Autodesk Inventor part; units mm, degrees
ref_plane "YZ Plane" through (0, 0, 0) normal (1, 0, 0) x (0, 1, 0)
ref_plane "XZ Plane" through (0, 0, 0) normal (0, 1, 0) x (-1, 0, 0)
ref_plane "XY Plane" through (0, 0, 0) normal (0, 0, 1) x (1, 0, 0)
sketch "スケッチ1" plane through (0, 0, 0) normal (0, 0, 1) x (1, 0, 0)
  circle A0 centre (-490.19, 90.19) radius 2.1
  circle A1 centre (-490.19, 290.19) radius 2.1
  circle A2 centre (-190.19, 390.19) radius 2.1
  circle A3 centre (-390.19, 390.19) radius 2.1
  circle A4 centre (-290.19, -9.81) radius 2.1
  circle A5 centre (-90.19, -9.81) radius 2.1
  circle A6 centre (9.81, 190.19) radius 2.1
  circle A7 centre (9.81, 390.19) radius 2.1
  circle A8 centre (-490.19, -9.81) radius 2.1
  circle A9 centre (-233.68, 12.7) radius 1.6 construction
  circle A10 centre (-29.21, 294.64) radius 1.6 construction
  circle A11 centre (-161.29, 294.64) radius 1.6 construction
  circle A12 centre (-233.68, 294.64) radius 1.6 construction
  circle A13 centre (-233.68, 137.16) radius 1.6 construction
  circle A14 centre (-161.29, 137.16) radius 1.6 construction
  circle A15 centre (-6.35, 137.16) radius 1.6 construction
  circle A16 centre (-6.35, 12.7) radius 1.6 construction
  circle A17 centre (-161.29, 12.7) radius 1.6 construction
  circle A18 centre (9.81, -9.81) radius 2.1
  circle A19 centre (-490.19, 390.19) radius 2.1
  circle A20 centre (9.81, 290.19) radius 2.1
  circle A21 centre (9.81, 90.19) radius 2.1
  circle A22 centre (-190.19, -9.81) radius 2.1
  circle A23 centre (-390.19, -9.81) radius 2.1
  circle A24 centre (-290.19, 390.19) radius 2.1
  circle A25 centre (-90.19, 390.19) radius 2.1
  circle A26 centre (-490.19, 190.19) radius 2.1
  line L0 (-21.19, 1.19) -> (-459.19, 1.19)
  line L1 (-479.19, 21.19) -> (-479.19, 359.19)
  line L2 (-459.19, 379.19) -> (-21.19, 379.19)
  line L3 (-1.19, 359.19) -> (-1.19, 21.19)
  circle A27 centre (9.81, -9.81) radius 5
  circle A28 centre (9.81, -9.81) radius 15.5563 construction
  line L4 (9.81, -9.81) -> (-1.19, 1.19) construction
  line L5 (9.81, -9.81) -> (25.3663, -9.81) construction
  circle A29 centre (-1.19, 1.19) radius 5 construction
  circle A30 centre (-1.19, 1.19) radius 2.1
  line L6 (-240.19, 1.19) -> (-240.19, 379.19) construction
  line L7 (-1.19, 190.19) -> (-479.19, 190.19) construction
  circle A31 centre (-1.19, 379.19) radius 2.1
  circle A32 centre (-479.19, 1.19) radius 2.1
  circle A33 centre (-479.19, 379.19) radius 2.1
  arc A34 (-1.19, 359.19) -> (-21.19, 379.19) centre (-21.19, 359.19) ccw
  arc A35 (-459.19, 379.19) -> (-479.19, 359.19) centre (-459.19, 359.19) ccw
  arc A36 (-479.19, 21.19) -> (-459.19, 1.19) centre (-459.19, 21.19) ccw
  arc A37 (-21.19, 1.19) -> (-1.19, 21.19) centre (-21.19, 21.19) ccw
  line L8 (9.81, -4.81) -> (-11.2166, -4.81) construction
  arc A38 (-483.7257, 425.19) -> (-483.7257, -44.81) centre (161.4767, 190.19) ccw
  line L9 (-483.7257, 425.19) -> (-379.99, 425.19)
  arc A39 (-379.99, 425.19) -> (-100.39, 425.19) centre (-240.19, 735.924) ccw
  line L10 (-100.39, 425.19) -> (3.3457, 425.19)
  arc A40 (3.3457, -44.81) -> (3.3457, 425.19) centre (-641.8567, 190.19) ccw
  line L11 (3.3457, -44.81) -> (-79.99, -44.81)
  arc A41 (-79.99, -44.81) -> (-400.39, -44.81) centre (-240.19, -457.544) ccw
  line L12 (-400.39, -44.81) -> (-483.7257, -44.81)
  arc A42 (14.81, 390.19) -> (9.81, 395.19) centre (9.81, 390.19) ccw
  line L13 (9.81, 395.19) -> (-490.19, 395.19)
  line L14 (14.81, -9.81) -> (14.81, 390.19)
  arc A43 (9.81, -14.81) -> (14.81, -9.81) centre (9.81, -9.81) ccw construction
  line L15 (-490.19, -14.81) -> (9.81, -14.81)
  arc A44 (-495.19, -9.81) -> (-490.19, -14.81) centre (-490.19, -9.81) ccw
  line L16 (-495.19, 390.19) -> (-495.19, -9.81)
  arc A45 (-490.19, 395.19) -> (-495.19, 390.19) centre (-490.19, 390.19) ccw
  point P0 (0, 0)
  point P1 (-1.19, 1.19)
  point P2 (-479.19, 379.19)
  point P3 (-479.19, 1.19)
  point P4 (-1.19, 379.19)
  point P5 (14.59, -11.277)
  point P6 (-494.97, 391.657)
  point P7 (-494.97, -11.277)
  dimension "d4" = 31.1127
  dimension "d5" = 135
  dimension "d6" = 10
  dimension "d10" = 20
  dimension "d11" = 6
  dimension "d14" = 11
  dimension "d15" = 11
  dimension "d16" = 11
  dimension "d17" = 11
  dimension "d18" = 11
  dimension "d30" = 100
extrude "押し出し1" add sketch "スケッチ1" against normal blind 3 contours A27 | A27 L15 A44 L16 A45 L13 A42 L14 | A27 A40 L11 A41 L15 | A41 L12 A38 A44 L15 | A30 | A32
sketch "スケッチ3" plane through (0, 0, -3) normal (0, 0, -1) x (-1, 0, 0)
  arc A0 (-14.81, -9.81) -> (-14.59, -11.277) centre (-9.81, -9.81) ccw
  arc A1 (-14.59, -11.277) -> (-3.3457, -44.81) centre (641.8567, 190.19) ccw
  arc A2 (483.7257, -44.81) -> (494.97, -11.277) centre (-161.4767, 190.19) ccw
  arc A3 (494.97, -11.277) -> (495.19, -9.81) centre (490.19, -9.81) ccw
  line L0 (-14.81, -9.81) -> (-14.81, -39.81)
  arc A4 (-14.81, -39.81) -> (-9.81, -44.81) centre (-9.81, -39.81) ccw
  line L1 (79.99, -44.81) -> (-3.3457, -44.81)
  line L2 (-9.81, -44.81) -> (-3.3457, -44.81)
  line L3 (495.19, -9.81) -> (495.19, -39.81)
  arc A5 (490.19, -44.81) -> (495.19, -39.81) centre (490.19, -39.81) ccw
  line L4 (490.19, -44.81) -> (483.7257, -44.81)
  point P0 (0, 0)
  dimension "d19" = 5
extrude "押し出し3" add sketch "スケッチ3" against normal up to surface (3 mm away)
fillet "フィレット2" radius 5 2 edges at (-79.99, -44.81, -1.5) (-400.39, -44.81, -1.5)
sketch "スケッチ4" plane through (0, 0, -3) normal (0, 0, -1) x (-1, 0, 0)
  arc A0 (-14.81, -39.81) -> (-9.81, -44.81) centre (-9.81, -39.81) ccw construction
  circle A1 centre (-9.81, -9.81) radius 2.1 construction
  arc A2 (490.19, -44.81) -> (495.19, -39.81) centre (490.19, -39.81) ccw construction
  circle A3 centre (490.19, -9.81) radius 2.1 construction
  line L0 (-9.81, -9.81) -> (1.19, 1.19) construction
  line L1 (1.19, 1.19) -> (1.19, -28.81) construction
  line L2 (1.19, -28.81) -> (-9.81, -39.81) construction
  line L3 (-9.81, -39.81) -> (-9.81, -9.81) construction
  line L4 (479.19, 1.19) -> (490.19, -9.81) construction
  line L5 (490.19, -9.81) -> (490.19, -39.81) construction
  line L6 (490.19, -39.81) -> (479.19, -28.81) construction
  line L7 (479.19, -28.81) -> (479.19, 1.19) construction
  circle A4 centre (-9.81, -39.81) radius 2.1
  circle A5 centre (490.19, -39.81) radius 2.1
  arc A6 (79.0564, -44.81) -> (80.8558, -44.475) centre (79.0564, -39.81) ccw construction
  arc A7 (399.5242, -44.475) -> (401.3236, -44.81) centre (401.3236, -39.81) ccw construction
  circle A8 centre (401.3236, -39.81) radius 2.1
  circle A9 centre (79.0564, -39.81) radius 2.1
  circle A10 centre (1.19, -28.81) radius 2.1
  circle A11 centre (479.19, -28.81) radius 2.1
  dimension "d27" = 11
  dimension "d28" = 11
  dimension "d29" = 45
extrude "押し出し4" cut sketch "スケッチ4" against normal through all
sketch "スケッチ5" plane through (0, 0, 0) normal (0, 0, 1) x (1, 0, 0)
  circle A0 centre (-490.19, 290.19) radius 2.1 construction
  circle A1 centre (-490.19, 190.19) radius 2.1 construction
  circle A2 centre (9.81, 90.19) radius 2.1 construction
  line L0 (9.81, 90.19) -> (9.81, 120.19) construction
  line L1 (-490.19, 290.19) -> (-490.19, 320.19) construction
  line L2 (-490.19, 190.19) -> (-490.19, 160.19) construction
  circle A3 centre (-490.19, 320.19) radius 2.1
  circle A4 centre (-490.19, 160.19) radius 2.1
  circle A5 centre (9.81, 120.19) radius 2.1
  circle A6 centre (9.81, 105.19) radius 2.1
  circle A7 centre (9.81, 135.19) radius 2.1
  circle A8 centre (-490.19, 175.19) radius 2.1
  dimension "d34" = 30
  dimension "d35" = 15
extrude "押し出し5" cut sketch "スケッチ5" against normal blind 30
equation "\"d35\" = 0.5 * d34"
equation "\"d32\" = d34"
properties part number "left_plate_01"
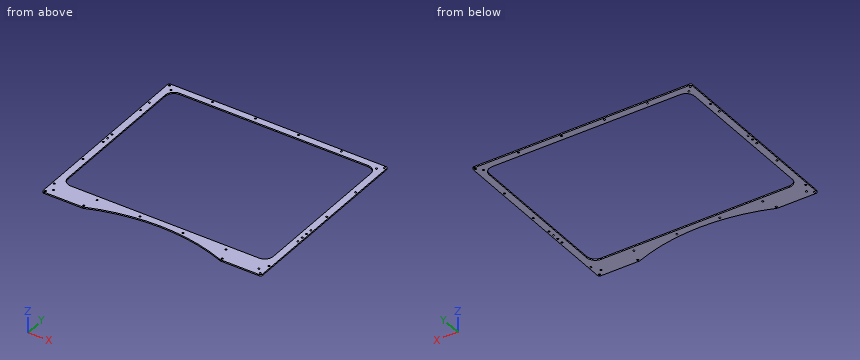
For this review, take the finished solid that the model builds, in its own axes (mm). Coordinates: 2 decimals unless noted, no trailing zeros. Loops run counter-clockwise (first coordinate to the right, second up) from the corner with the lowest first, then second, coordinate; pieces in that order, holes last. Notation, with made-up numbers: (32.5, 59.5) - (57.5, 59.5) arc R21 cw to (57.5, 64.5) - close; hole circle Ø11 at (-16, -2.5). An arc over 180 degrees is marked (long way). Use one line per item in the form item = value. Start each with the question number.
1) Take a section at B-B (x = -362.5). State the section outline as (y, z) points.
2) To check wall thickness, follow probe 1 along X at (y, z) = (266.5, -2.05); probe 2 along Y at (x, z) = (-90.19, -1.15); probe 3 along Y at (x, z) = (-37, -1.3). State the ranges of each line that lie inside material, in increasing order. Write a range as from..to.
3) Take a section at C-C (z = -1.7). State how many separate pieces and enclosed holes the cut face has, plus the area to 3 significant figures.
4) For pin 1 (1.5 mm diameter, centred on x = -112, z = -2.5, fed in from -Y), flat-tipped, find the tip position at first contact; note if it passes through.
5) Take a section at A-A (y = 232.5). State the section outline as (x, z) points, plus the area to 3 significant figures.
From the geometry:
q1.outline = (-32.04, -3) - (1.19, -3) - (1.19, 0) - (-32.04, 0) - close; (379.19, -3) - (395.19, -3) - (395.19, 0) - (379.19, 0) - close
q2.probe_1 = -495.19..-479.19, -1.19..14.81
q2.probe_2 = -40.99..-11.91, -7.71..1.19, 379.19..388.09, 392.29..395.19
q2.probe_3 = -44.81..1.19, 379.19..395.19
q3.separate_pieces = 1
q3.enclosed_holes = 33
q3.area = 37,100 mm2
q4.pin_1 = -34
q5.outline = (-495.19, -3) - (-479.19, -3) - (-479.19, 0) - (-495.19, 0) - close; (-1.19, -3) - (14.81, -3) - (14.81, 0) - (-1.19, 0) - close
q5.area = 96.0 mm2
